```python
from build123d import *

# Parameters (mm, degrees)
SKETCH2_R           = 2.625
SKETCH2_R_2         = 6.477
SKETCH2_R_3         = 2.4
SKETCH2_R_4         = 10
SKETCH2_R_5         = 4.5000037
BOSS_EXTRUDE1_DEPTH = 3.175
BOSS_EXTRUDE2_START = -3.175
BOSS_EXTRUDE2_DEPTH = 3.175
FILLET1_R           = 2.54


with BuildPart() as part:
    # Sketch2 → Boss-Extrude1 (new body)
    with BuildSketch(Plane.XY):
        with BuildLine():
            Line((-16.662660117, 125.372318995), (128.780651825, 125.372318995))
            ThreePointArc((128.780651825, 125.372318995), (133.270779886, 123.512447055), (135.130651825, 119.022318995))
            Line((135.130651825, 119.022318995), (135.130651825, -19.407679937))
            ThreePointArc((135.130651825, -19.407679937), (133.642754274, -22.999782385), (130.050651825, -24.487679937))
            Line((130.050651825, -24.487679937), (17.627339883, -24.487679937))
            ThreePointArc((17.627339883, -24.487679937), (-11.109479704, -12.584499524), (-23.012660117, 16.152320063))
            Line((-23.012660117, 16.152320063), (-23.012660117, 119.022318995))
            ThreePointArc((-23.012660117, 119.022318995), (-21.152788178, 123.512447055), (-16.662660117, 125.372318995))
        make_face()
        with Locations((-14.122660117, 115.657274828)):
            Circle(SKETCH2_R, mode=Mode.SUBTRACT)
        with Locations((56.050128961, 79.792333504)):
            Circle(SKETCH2_R_2, mode=Mode.SUBTRACT)
        with Locations((56.034611898, 62.012340275)):
            Circle(SKETCH2_R_3, mode=Mode.SUBTRACT)
        with Locations((56.067862747, 100.112325766)):
            Circle(SKETCH2_R_2, mode=Mode.SUBTRACT)
        with Locations((56.08337981, 117.892318995)):
            Circle(SKETCH2_R_3, mode=Mode.SUBTRACT)
        with Locations((36.9797887, 56.4940647)):
            Circle(SKETCH2_R_2, mode=Mode.SUBTRACT)
        with Locations((39.880571418, 115.657274828)):
            Circle(SKETCH2_R, mode=Mode.SUBTRACT)
        with Locations((74.777420291, 115.710615977)):
            Circle(SKETCH2_R, mode=Mode.SUBTRACT)
        with Locations((-14.122660117, 50.442319529)):
            Circle(SKETCH2_R, mode=Mode.SUBTRACT)
        with Locations((-5.124288877, -6.016277999)):
            Circle(SKETCH2_R, mode=Mode.SUBTRACT)
        with Locations((73.296411889, -15.597679937)):
            Circle(SKETCH2_R, mode=Mode.SUBTRACT)
        with Locations((126.240651825, 15.946756738)):
            Circle(SKETCH2_R, mode=Mode.SUBTRACT)
        with Locations((11.5011229, 89.92565906)):
            Circle(SKETCH2_R_4, mode=Mode.SUBTRACT)
        with Locations((100.509036058, 89.97900021)):
            Circle(SKETCH2_R_4, mode=Mode.SUBTRACT)
        with Locations((88.617464572, 104.15082325)):
            Circle(SKETCH2_R_5, mode=Mode.SUBTRACT)
        with Locations((112.400607544, 75.80717717)):
            Circle(SKETCH2_R_5, mode=Mode.SUBTRACT)
        with Locations((-0.390448587, 104.097482101)):
            Circle(SKETCH2_R_5, mode=Mode.SUBTRACT)
        with Locations((23.518543133, 75.859913549)):
            Circle(SKETCH2_R_5, mode=Mode.SUBTRACT)
    extrude(amount=BOSS_EXTRUDE1_DEPTH)

    # Sketch3 → Boss-Extrude2 (add)
    with BuildSketch(Plane.XY.offset(3.175).offset(BOSS_EXTRUDE2_START)):
        with BuildLine():
            Line((-23.012660117, 119.022318995), (-23.012660117, 144.422318995))
            Line((-23.012660117, 144.422318995), (135.130651825, 144.422318995))
            Line((135.130651825, 144.422318995), (135.130651825, 119.022318995))
            ThreePointArc((135.130651825, 119.022318995), (133.270779886, 123.512447055), (128.780651825, 125.372318995))
            Line((128.780651825, 125.372318995), (-16.662660117, 125.372318995))
            ThreePointArc((-16.662660117, 125.372318995), (-21.152788178, 123.512447055), (-23.012660117, 119.022318995))
        make_face()
    extrude(amount=BOSS_EXTRUDE2_DEPTH)

    # Fillet1
    fillet1_edges = [part.edges().sort_by_distance(p)[0] for p in [
        (-23.012660117, 144.422318995, 1.5875),
        (135.130651825, 144.422318995, 1.5875),
    ]]
    fillet(fillet1_edges, radius=FILLET1_R)


solid = part.part
```
Part model, mm, in its own coordinate system. Round coordinates to 2 decimals unless told otherwise and drop trailing zeros. Loops run counter-clockwise (first coordinate to the right, second up) from the corner with the lowest first, then second, coordinate; pieces in that order, holes last.
1. Flat gauge pin, fed straight in: pin 1 (4 mm diameter, centred on x = 56.03, y = 62.01, fed in from +Z). Where does the tip first touch, or does it go through?
Solutions:
pin 1: passes through
2. Drill centre lines: line 1 along X through (y, z) = (114.5, 1); line 2 along X through (y, z) = (92, 0.85); line 3 along Y through (x, z) = (-14, 2.05). Where is each one in solid material? Low to high.
Solutions:
line 1: x = -23.01 to -16.48, -11.77 to 37.52, 42.24 to 72.45, 77.11 to 135.13
line 2: x = -23.01 to 1.72, 21.28 to 90.72, 110.3 to 135.13
line 3: y = -9.37 to 47.82, 53.06 to 113.04, 118.28 to 144.42
3. Two-plate mould, pull along Y, no slides. Class faces 1 (the face through (133.68, -22.96, 1.57)), 2 (the face through (57.14, 59.88, 1.57)), 3 (the face through (75, 61, 3.175)): pulls with the +Y half, pulls with the -Y half, needs draft (parallel to the pull), parting line crosses it, or undercut.
Solutions:
face 1: pulls with the -Y half
face 2: undercut
face 3: needs draft
4. Slice it at B-B (y = 95.5). Give the cut face in (x, z) (3 decimals), and give its area (3 significant figures).
Solutions:
outline: (-23.013, 0) - (3.199, 0) - (3.199, 3.175) - (-23.013, 3.175) - close; (19.803, 0) - (51.521, 0) - (51.521, 3.175) - (19.803, 3.175) - close; (60.615, 0) - (92.171, 0) - (92.171, 3.175) - (60.615, 3.175) - close; (108.847, 0) - (135.131, 0) - (135.131, 3.175) - (108.847, 3.175) - close
area: 368 mm2
5. Slice it at A-A (x = 115). Give the cut face in (y, z) (3 decimals), and give its area (3 significant figures).
Solutions:
outline: (-24.488, 0) - (72.134, 0) - (72.134, 3.175) - (-24.488, 3.175) - close; (79.48, 0) - (144.422, 0) - (144.422, 3.175) - (79.48, 3.175) - close
area: 513 mm2
6. Slice it at D-D (x = 23.5). Give the cut face in (y, z) (3 decimals).
Solutions:
outline: (-24.488, 0) - (71.36, 0) - (71.36, 3.175) - (-24.488, 3.175) - close; (80.36, 0) - (144.422, 0) - (144.422, 3.175) - (80.36, 3.175) - close
7. Slice it at C-C (z = 2.25). Count the separate pieces of the cut face and the enclosed holes in it, and give its area (3 significant figures).
Solutions:
separate pieces: 1
enclosed holes: 18
area: 24,900 mm2
